Build history of the part. All positions in model axes, mm. A direction names the side the tool comes from. Give positions to 0.01 mm unless a question says otherwise; leave off trailing zeros. Order: outer loops, then holes, each group sorted by start corner. A loop starts at its lowest first (then second) coordinate and runs counter-clockwise, first axis right, second up. Notation, with made-up numbers: M 73,-27.5 L 94,-27.5 A8 ccw 94,-23.5 Z; hole C 72,-29.5 d5. An arc over 180 degrees is marked long. One line per item, written item: value.
Autodesk Inventor part; units mm, degrees
ref_plane "YZ Plane" through (0, 0, 0) normal (1, 0, 0) x (0, 1, 0)
ref_plane "XZ Plane" through (0, 0, 0) normal (0, 1, 0) x (-1, 0, 0)
ref_plane "XY Plane" through (0, 0, 0) normal (0, 0, 1) x (1, 0, 0)
sketch "Szkic1" plane through (0, 0, 0) normal (0, 0, 1) x (1, 0, 0)
  line L0 (-10.699, 18.8462) -> (5.301, 18.8462)
  line L1 (5.301, 18.8462) -> (5.301, -13.5538)
  line L2 (5.301, -13.5538) -> (-10.699, -13.5538)
  line L3 (-10.699, -13.5538) -> (-10.699, 18.8462)
  point P0 (0, 0)
  dimension "d0" = 16
  dimension "d1" = 32.4
extrude "Wyciągnięcie proste1" add sketch "Szkic1" along normal blind 12
sketch "Szkic2" plane through (-10.699, -13.5538, 0) normal (-1, 0, 0) x (0, 0, 1)
  line L0 (0, 0) -> (0, 32.4)
  line L1 (0, 0) -> (12, 0)
  line L2 (12, 32.4) -> (12, 0)
  line L3 (0, 32.4) -> (12, 32.4)
  line L4 (12, 32.4) -> (12, 0)
  circle A0 centre (12.2, 16.2) radius 6.05
  point P0 (0, 13.5538)
  dimension "d4" = 32.4
  dimension "d6" = 12.1
  dimension "d66" = 16.2
  dimension "d67" = 0.2
extrude "Wyciągnięcie proste2" cut sketch "Szkic2" against normal blind 13 contours A0 L2 | L2 A0
sketch "Szkic3" plane through (-10.699, -13.5538, 0) normal (-1, 0, 0) x (0, 0, 1)
  arc A0 (12, 22.2467) -> (12, 10.1533) centre (12.2, 16.2) ccw
  line L0 (12, 32.4) -> (12, 22.2467)
  line L1 (0, 32.4) -> (12, 32.4)
  line L2 (0, 0) -> (0, 32.4)
  line L3 (0, 0) -> (12, 0)
  line L4 (12, 10.1533) -> (12, 0)
  arc A1 (12, 24.2725) -> (12, 8.1275) centre (12.2, 16.2) ccw
  point P0 (0, 13.5538)
  dimension "d9" = 16.15
extrude "Wyciągnięcie proste3" cut sketch "Szkic3" against normal blind 7.15 contours A0 L4 A1 L0
extrude "Wyciągnięcie proste4" add sketch "Szkic3" against normal blind 3.3 contours A0 L4 A1 L0
sketch "Szkic6" plane through (5.301, -13.5538, 0) normal (1, 0, 0) x (0, 0, -1)
  arc A0 (-12, 8.1275) -> (-12, 24.2725) centre (-12.2, 16.2) ccw
  line L0 (0, 32.4) -> (0, 0)
  line L1 (0, 32.4) -> (-12, 32.4)
  line L2 (-12, 0) -> (-12, 32.4)
  line L3 (0, 0) -> (-12, 0)
  arc A1 (-12, 8.1275) -> (-12, 24.2725) centre (-12.2, 16.2) ccw
  point P0 (0, 13.5538)
extrude "Wyciągnięcie proste5" cut sketch "Szkic6" against normal blind 3.15 contours L2 A0
sketch "Szkic7" plane through (0, 0, 12) normal (0, 0, 1) x (1, 0, 0)
  line L0 (5.301, -5.4264) -> (2.151, -5.4264)
  line L1 (2.151, -5.4264) -> (2.151, -3.4005)
  line L2 (2.151, -3.4005) -> (-3.549, -3.4005)
  line L3 (-3.549, -3.4005) -> (-3.549, -5.4264)
  line L4 (-3.549, -5.4264) -> (-7.399, -5.4264)
  line L5 (-7.399, -3.4005) -> (-7.399, -5.4264)
  line L6 (-10.699, -3.4005) -> (-7.399, -3.4005)
  line L7 (-10.699, -3.4005) -> (-10.699, -13.5538)
  line L8 (-10.699, -13.5538) -> (5.301, -13.5538)
  line L9 (5.301, -13.5538) -> (5.301, -5.4264)
  line L10 (2.151, 10.7187) -> (5.301, 10.7187)
  line L11 (5.301, 10.7187) -> (5.301, 18.8462)
  line L12 (5.301, 18.8462) -> (-10.699, 18.8462)
  line L13 (-10.699, 18.8462) -> (-10.699, 8.6929)
  line L14 (-10.699, 8.6929) -> (-7.399, 8.6929)
  line L15 (-7.399, 10.7187) -> (-7.399, 8.6929)
  line L16 (-7.399, 10.7187) -> (-3.549, 10.7187)
  line L17 (-3.549, 10.7187) -> (-3.549, 8.6929)
  line L18 (-3.549, 8.6929) -> (2.151, 8.6929)
  line L19 (2.151, 8.6929) -> (2.151, 10.7187)
  point P0 (0, 0)
  point P1 (-0.699, -7.3538)
  point P2 (-0.699, 12.6462)
  dimension "d46" = 20
  dimension "d47" = 32.4
  dimension "d48" = 6.2
  dimension "d49" = 6.2
  dimension "d50" = 5.7
  dimension "d68" = 10
  dimension "d69" = 10
hole "Otwór3" at (-0.699, -7.3538, 12) at (-0.699, 12.6462, 12) direction (0, 0, -1) diameter 3 end through all
sketch "Szkic8" plane through (-10.699, -13.5538, 0) normal (-1, 0, 0) x (0, 0, 1)
  line L0 (12, 32.4) -> (12, 22.2467)
  line L1 (0, 32.4) -> (12, 32.4)
  line L2 (0, 0) -> (0, 32.4)
  line L3 (0, 0) -> (12, 0)
  line L4 (12, 10.1533) -> (12, 0)
  arc A0 (12, 22.2467) -> (12, 10.1533) centre (12.2, 16.2) ccw
  point P0 (0, 13.5538)
extrude "Wyciągnięcie proste6" add sketch "Szkic8" along normal blind 2
chamfer "Faza4" distance 1 angle 45 1 edges at (-12.699, 2.6462, 6.15)
chamfer "Faza5" distance 1.5 angle 45 4 edges at (-12.699, 18.8462, 6) (5.301, 18.8462, 6) (-12.699, -13.5538, 6) (5.301, -13.5538, 6)
sketch "Szkic9" plane through (0, 0, 12) normal (0, 0, 1) x (1, 0, 0)
  line L0 (5.301, -12.0538) -> (3.801, -13.5538)
  line L1 (5.301, -12.0538) -> (5.301, -5.4264)
  line L2 (5.301, -5.4264) -> (2.151, -5.4264)
  line L3 (2.151, -5.4264) -> (2.151, -3.4005)
  line L4 (2.151, -3.4005) -> (-3.549, -3.4005)
  line L5 (-3.549, -3.4005) -> (-3.549, -5.4264)
  line L6 (-3.549, -5.4264) -> (-7.399, -5.4264)
  line L7 (-7.399, -3.4005) -> (-7.399, -5.4264)
  line L8 (-11.699, -3.4005) -> (-7.399, -3.4005)
  line L9 (-12.699, -12.0538) -> (-12.699, -4.401)
  line L10 (-11.199, -13.5538) -> (-12.699, -12.0538)
  line L11 (3.801, -13.5538) -> (-11.199, -13.5538)
  circle A0 centre (-0.699, -7.3538) radius 1.5
  line L12 (3.801, 18.8462) -> (5.301, 17.3462)
  line L13 (3.801, 18.8462) -> (-11.199, 18.8462)
  line L14 (-12.699, 17.3462) -> (-11.199, 18.8462)
  line L15 (-12.699, 9.6933) -> (-12.699, 17.3462)
  line L16 (-7.399, 8.6929) -> (-11.699, 8.6929)
  line L17 (-7.399, 10.7187) -> (-7.399, 8.6929)
  line L18 (-7.399, 10.7187) -> (-3.549, 10.7187)
  line L19 (-3.549, 10.7187) -> (-3.549, 8.6929)
  line L20 (-3.549, 8.6929) -> (2.151, 8.6929)
  line L21 (2.151, 8.6929) -> (2.151, 10.7187)
  line L22 (2.151, 10.7187) -> (5.301, 10.7187)
  line L23 (5.301, 10.7187) -> (5.301, 17.3462)
  circle A1 centre (-0.699, 12.6462) radius 1.5
  point P0 (0, 0)
  point P1 (-9.199, -9.5538)
  point P2 (-9.199, 14.8462)
  dimension "d78" = 3.5
  dimension "d79" = 3.5
  dimension "d80" = 4
  dimension "d81" = 4
hole "Otwór4" at (-9.199, -9.5538, 12) at (-9.199, 14.8462, 12) direction (0, 0, -1) diameter 2.6 end through all
properties part number "3DP_ABS_E3D_V6_Mount_Clamp"
1) Tool access for faces 1 (the face through (-3.549, 3, 6)), 2 (the face through (-11.938, 18.107, 5.916)), 3 (the face through (2.151, 3, 5)): list every direction of +Z, -Z, +X, -X, +Y, -Y with a clear straight run to the whole face (end or side of a thin tool).
Check values:
face 1: +Z
face 2: +Z, -Z, -X, +Y
face 3: +Z, +X
2) Saw through at A-A, the plane y = 15. Write the cut outline in (x, z), then the cut area to 3 significant figures.
Check values:
outline: M -12.7,0 L -10.49,0 L -10.49,12 L -12.7,12 Z; M -7.91,0 L 5.3,0 L 5.3,12 L -7.91,12 Z
area: 185 mm^2
3) Drill centre lines: probe 1 along Y at (x, z) = (-10, 11.5); probe 2 along Y at (x, z) = (-2, 10.25); probe 3 along X at (y, z) = (-8.5, 3.25). Where is each one in solid material? Low to high. Write a range as from..to.
Check values:
probe 1: -13.55..-10.58, -8.53..-3.36, 8.66..13.82, 15.87..18.85
probe 2: -13.55..-8.1, -6.61..-3.08, 8.37..11.9, 13.39..18.85
probe 3: -12.7..-9.96, -8.44..-1.67, 0.27..5.3
4) Pin check, flat tips, straight feed: pin 1 (10 mm diameter, centred on x = 2, y = 2.5, fed in from +Z); pin 2 (4 mm diameter, centred on y = 2.5, z = 7.5, fed in from +X). Stop position of each tip, or through.
Check values:
pin 1: z = 9.02
pin 2: x = 2.15
5) Saw through at C-C, the plane x = -0.25. Write the cut outline in (y, z), then the cut area to 3 significant figures.
Check values:
outline: M -13.55,0 L -8.79,0 L -8.79,12 L -13.55,12 Z; M -5.92,0 L 11.21,0 L 11.21,12 L 8.69,12 A6.05 cw -3.4,12 L -5.92,12 Z; M 14.08,0 L 18.85,0 L 18.85,12 L 14.08,12 Z
area: 265 mm^2
6) Mould opens along Y. For faces 4 (the face through (3.748, 2.471, 4.127)), 5 (the face through (-4, 2, 0)), 6 (the face through (-4, -13.554, 6)) say: released by +Y, released by -Y, zero draft, split by the parting line, or undercut.
Check values:
face 4: undercut
face 5: zero draft
face 6: released by -Y
7) Saw through at B-B, the plane z = 2. Write the cut outline in (x, y), then the cut area to 3 significant figures.
Check values:
outline: M -12.7,-12.05 L -11.2,-13.55 L 3.8,-13.55 L 5.3,-12.05 L 5.3,17.35 L 3.8,18.85 L -11.2,18.85 L -12.7,17.35 Z; hole C -9.2,-9.55 d2.6; hole C -9.2,14.85 d2.6; hole C -0.7,-7.35 d3; hole C -0.7,12.65 d3
area: 554 mm^2
